Here's how the part is built. I have some questions about the finished solid (model axes, mm). Face numbers are marked on the shaded views. A direction names the side the tool comes from. Give positions to 0.01 mm unless a question says otherwise; leave off trailing zeros. Write each loop counter-clockwise with the first axis right and the second up, starting at its lowest first coordinate (ties: lowest second). Pieces come first, ordered by that corner, then holes. Notation, with made-up numbers: (77.5, 50) - (133.5, 50) arc R20 ccw to (133.5, 72) - close; hole circle Ø2 at (72, -17.5). An arc over 180 degrees is marked (long way). One line per item, written item: value. Start each with the question number.
1) We'd pull the mould along Y, two halves only. Please class the marked faces 3 and 4: +Y half, -Y half, draft (parallel to the pull), parting line (faces both ways), or undercut.
2) Please list where these lines run through material, in increasing order: L1, parallel to Y at x = 8.5, z = 1; L2, parallel to Z at x = -7, y = -13.5; L3, parallel to Z at x = 7, y = -2. Write a range as [from, to].
3) Imagine slicing it at D-D on x = -4. Write out the boundary of the cut face in (y, z).
4) Imagine slicing it at C-C on z = 21.5. Write out the boundary of the cut face in (x, y).
5) I'm going to push flat-ended pins straight in: P1, Ø5, axis at x = 2, z = 29, coming from the +Y side; P2, Ø5, axis at x = 8, y = -3.5, coming from the -Z side; P3, Ø12, axis at x = -7, z = -2, coming from the -Y side; P4, Ø4, axis at y = 2.5, z = -5, coming from the -X side. Where does each tip first touch, or does it pass through?
6) On a 3-axis mill with a long thin cutter (end or side, diameter ignored), from which of +Z, -Z, +X, -X, +Y, -Y can I reach the whole of each face in a straight line? I mean the marked faces 1 and 2. Say none if no direction works.
7) Imagine slicing it at A-A on x = 0. Write out the boundary of the cut face in (y, z).
8) Imagine slicing it at B-B on y = 0. Write out the boundary of the cut face in (x, z).
from build123d import *

# Parameters (mm, degrees)
SKETCH1_R           = 18.5
BOSS_EXTRUDE1_DEPTH = 70
SKETCH2_R           = 5.969
BOSS_EXTRUDE2_DEPTH = 6.096
SKETCH3_R           = 3.048
BOSS_EXTRUDE3_DEPTH = 16.002
SKETCH4_R           = 1.6
CUT_EXTRUDE1_DEPTH  = 3
SKETCH5_W           = 4.032124998
SKETCH5_H           = 0.762
CUT_EXTRUDE2_DEPTH  = 16.002


with BuildPart() as part:
    # Sketch1 → Boss-Extrude1 (new body)
    with BuildSketch(Plane.XY):
        Circle(SKETCH1_R)
    extrude(amount=BOSS_EXTRUDE1_DEPTH)

    # Sketch2 → Boss-Extrude2 (add)
    with BuildSketch(Plane(origin=(0, 0, 0), x_dir=(-1, 0, 0), z_dir=(0, 0, -1))):
        with Locations((0, -7.112)):
            Circle(SKETCH2_R)
    extrude(amount=BOSS_EXTRUDE2_DEPTH)

    # Sketch3 → Boss-Extrude3 (add)
    with BuildSketch(Plane(origin=(0, 0, -6.096), x_dir=(-1, 0, 0), z_dir=(0, 0, -1))):
        with Locations((0, -7.112)):
            Circle(SKETCH3_R)
    extrude(amount=BOSS_EXTRUDE3_DEPTH)

    # Sketch4 → Cut-Extrude1 (cut)
    with BuildSketch(Plane(origin=(0, 0, 0), x_dir=(-1, 0, 0), z_dir=(0, 0, -1))):
        with Locations((-15.2766, 0)):
            Circle(SKETCH4_R)
        with Locations((15.2766, 0)):
            Circle(SKETCH4_R)
        with Locations((7.794229315, -13.567540858)):
            Circle(SKETCH4_R)
        with Locations((-7.794229315, -13.567540858)):
            Circle(SKETCH4_R)
        with Locations((-7.794229315, 13.214096537)):
            Circle(SKETCH4_R)
        with Locations((7.794229315, 13.214096537)):
            Circle(SKETCH4_R)
    extrude(amount=-CUT_EXTRUDE1_DEPTH, mode=Mode.SUBTRACT)

    # Sketch5 → Cut-Extrude2 (cut)
    with BuildSketch(Plane(origin=(0, 0, -22.098), x_dir=(-1, 0, 0), z_dir=(0, 0, -1))):
        with Locations((0, -4.445)):
            Rectangle(SKETCH5_W, SKETCH5_H)
    extrude(amount=-CUT_EXTRUDE2_DEPTH, mode=Mode.SUBTRACT)


solid = part.part
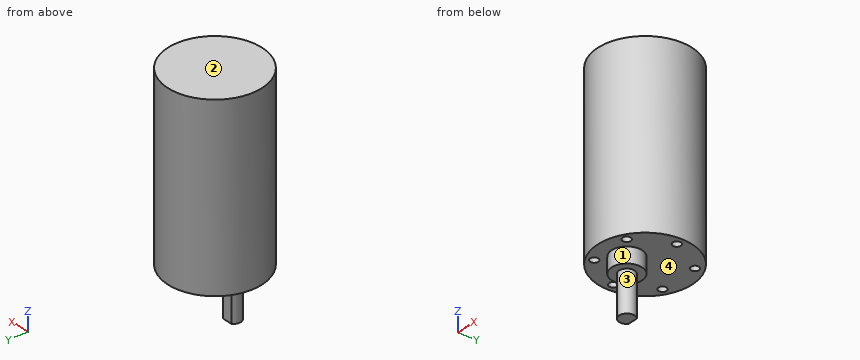
Numbers:
1. face 3: parting line
1. face 4: draft
2. L1: [-16.43, -15], [-12.13, 11.78], [14.65, 16.43]
2. L2: [3, 70]
2. L3: [0, 70]
3. outline: (-18.06, 0) - (-11.54, 0) - (-11.54, -6.1) - (-2.68, -6.1) - (-2.68, 0) - (18.06, 0) - (18.06, 70) - (-18.06, 70) - close
4. outline: circle Ø37 at (0, 0)
5. P1: y = 18.5
5. P2: z = 0
5. P3: y = -18.45
5. P4: through
6. face 1: -Z
6. face 2: +Z, +X, -X, +Y, -Y
7. outline: (-18.5, 0) - (-13.08, 0) - (-13.08, -6.1) - (-10.16, -6.1) - (-10.16, -22.1) - (-4.83, -22.1) - (-4.83, -6.1) - (-1.14, -6.1) - (-1.14, 0) - (18.5, 0) - (18.5, 70) - (-18.5, 70) - close
8. outline: (-18.5, 0) - (-16.88, 0) - (-16.88, 3) - (-13.68, 3) - (-13.68, 0) - (13.68, 0) - (13.68, 3) - (16.88, 3) - (16.88, 0) - (18.5, 0) - (18.5, 70) - (-18.5, 70) - close
